Geometry check sheet. Reference: the model listing, model coordinates, mm. Give positions to 0.01 mm unless a question says otherwise; leave off trailing zeros. Write each loop counter-clockwise with the first axis right and the second up, starting at its lowest first coordinate (ties: lowest second). Pieces come first, ordered by that corner, then holes. Notation, with made-up numbers: M 41.5,72.5 L 48.5,72.5 A15 ccw 48.5,82.5 Z; hole C 40,-13.5 d7. An arc over 180 degrees is marked long. One line per item, written item: value. Start each with the question number.
1. Cross-section at A-A on y = -2. Record the cut outline in (x, z), then the cut area to 3 significant figures.
2. Cross-section at C-C on x = 23. Record the cut outline in (y, z), then the cut area to 3 significant figures.
3. Gauge pin test, flat ends, axial feed: pin 1 (4 mm diameter, centred on x = 86.5, z = 4, fed in from +Y); pin 2 (5 mm diameter, centred on y = 6, z = 6.5, fed in from -X); pin 3 (1 mm diameter, centred on x = 22.5, z = 1.5, fed in from +Y); pin 4 (1.5 mm diameter, centred on x = -95, z = 4.5, fed in from -Y). Record the tip position at first contact, or that the pin passes through.
4. Cross-section at B-B on y = 7.5. Count the separate pieces of the cut face and the enclosed holes in it, then the cut area to 3 significant figures.
5. Scan lines: line 1 (Y direction, x = 67.5, z = 8); line 2 (X direction, y = -3.5, z = 2.25); line 3 (Y direction, x = 84, z = 7). Record each from-to range of solid material in increasing order.
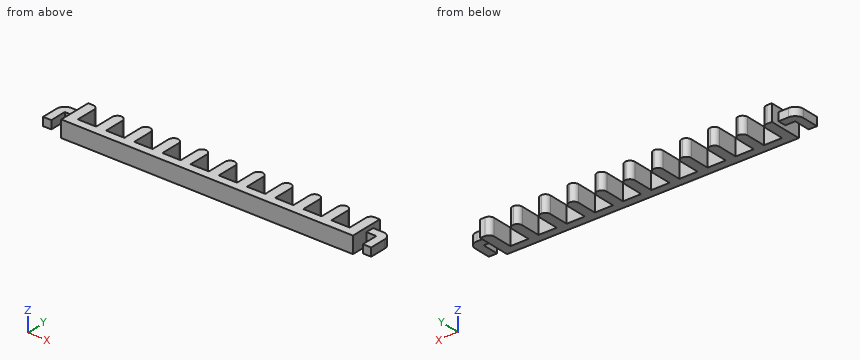
from build123d import *

# Parameters (mm, degrees)
F1_DEPTH  = 10
F2_W      = 5
F2_H      = 5
F3_DEPTH  = 11
F4_W      = 5
F4_H      = 5
F5_DEPTH  = 10
F6_R      = 2.99999
F7_R      = 5
F8_W      = 5
F8_H      = 5
F9_DEPTH  = 11
F10_W     = 5
F10_H     = 5
F11_DEPTH = 10
F12_R     = 5


# Not quite as in the source:
# - a fillet or chamfer is up to 0.001 mm smaller than in the source, because OpenCascade refuses the exact size


with BuildPart() as f1:
    # F0 (on Top) → F1 (new body)
    with BuildSketch(Plane.XY):
        Polygon((83, -5), (83, 15), (77, 15), (77, 0), (66, 0), (66, 15), (60, 15), (60, 0), (49, 0), (49, 15), (43, 15), (43, 0), (32, 0), (32, 15), (26, 15), (26, 0), (15, 0), (15, 15), (9, 15), (9, 0), (-2, 0), (-2, 15), (-8, 15), (-8, 0), (-19, 0), (-19, 15), (-25, 15), (-25, 0), (-36, 0), (-36, 15), (-42, 15), (-42, 0), (-53, 0), (-53, 15), (-59, 15), (-59, 0), (-70, 0), (-70, 15), (-76, 15), (-76, 0), (-87, 0), (-87, 15), (-93, 15), (-93, -5), align=None)
    extrude(amount=F1_DEPTH)

    # F2 (on face) → F3 (join)
    with BuildSketch(Plane(origin=(-93, 0, 0), x_dir=(0, -1, 0), z_dir=(-1, 0, 0))):
        with Locations((-7.5, 5)):
            Rectangle(F2_W, F2_H)
    extrude(amount=F3_DEPTH)

    # F4 (on face) → F5 (join)
    with BuildSketch(Plane.XZ.offset(-5)):
        with Locations((-101.5, 5)):
            Rectangle(F4_W, F4_H)
    extrude(amount=F5_DEPTH)

    # F6 (radius 3 in the source; OpenCascade refuses exactly that, so slightly less here)
    f6_edges = [f1.edges().sort_by_distance(p)[0] for p in [
        (-87, 15, 5),
        (-76, 15, 5),
        (-70, 15, 5),
        (-59, 15, 5),
        (-53, 15, 5),
        (-42, 15, 5),
        (-36, 15, 5),
        (-25, 15, 5),
        (-19, 15, 5),
        (-8, 15, 5),
        (-2, 15, 5),
        (9, 15, 5),
        (15, 15, 5),
        (26, 15, 5),
        (32, 15, 5),
        (43, 15, 5),
        (49, 15, 5),
        (60, 15, 5),
        (66, 15, 5),
        (77, 15, 5),
    ]]
    fillet(f6_edges, radius=F6_R)

    # F7
    f7_edges = [f1.edges().sort_by_distance(p)[0] for p in [
        (-104, 10, 5),
    ]]
    fillet(f7_edges, radius=F7_R)

    # F8 (on face) → F9 (join)
    with BuildSketch(Plane.YZ.offset(83)):
        with Locations((7.5, 5)):
            Rectangle(F8_W, F8_H)
    extrude(amount=F9_DEPTH)

    # F10 (on face) → F11 (join)
    with BuildSketch(Plane.XZ.offset(-5)):
        with Locations((91.5, 5)):
            Rectangle(F10_W, F10_H)
    extrude(amount=F11_DEPTH)

    # F12
    f12_edges = [f1.edges().sort_by_distance(p)[0] for p in [
        (94, 10, 5),
    ]]
    fillet(f12_edges, radius=F12_R)


solid = f1.part
Report:
1. outline: M -104,2.5 L -99,2.5 L -99,7.5 L -104,7.5 Z; M -93,0 L 83,0 L 83,10 L -93,10 Z; M 89,2.5 L 94,2.5 L 94,7.5 L 89,7.5 Z
1. area: 1,810 mm^2
2. outline: M -5,0 L 0,0 L 0,10 L -5,10 Z
2. area: 50.0 mm^2
3. pin 1: stops at y = 10
3. pin 2: stops at x = -104
3. pin 3: stops at y = 0
3. pin 4: stops at y = 5
4. separate pieces: 11
4. enclosed holes: 0
4. area: 763 mm^2
5. line 1: y = -5 to 0
5. line 2: x = -93 to 83
5. line 3: y = 5 to 10
